Check sheet for the drawn part. Datum: minimum x, y, z corner. Units: mm. A direction names the side the tool comes from. Give positions to 0.01 mm unless a question says otherwise; leave off trailing zeros. Write each loop counter-clockwise with the first axis right and the second up, starting at its lowest first coordinate (ties: lowest second). Pieces come first, ordered by that corner, then holes.
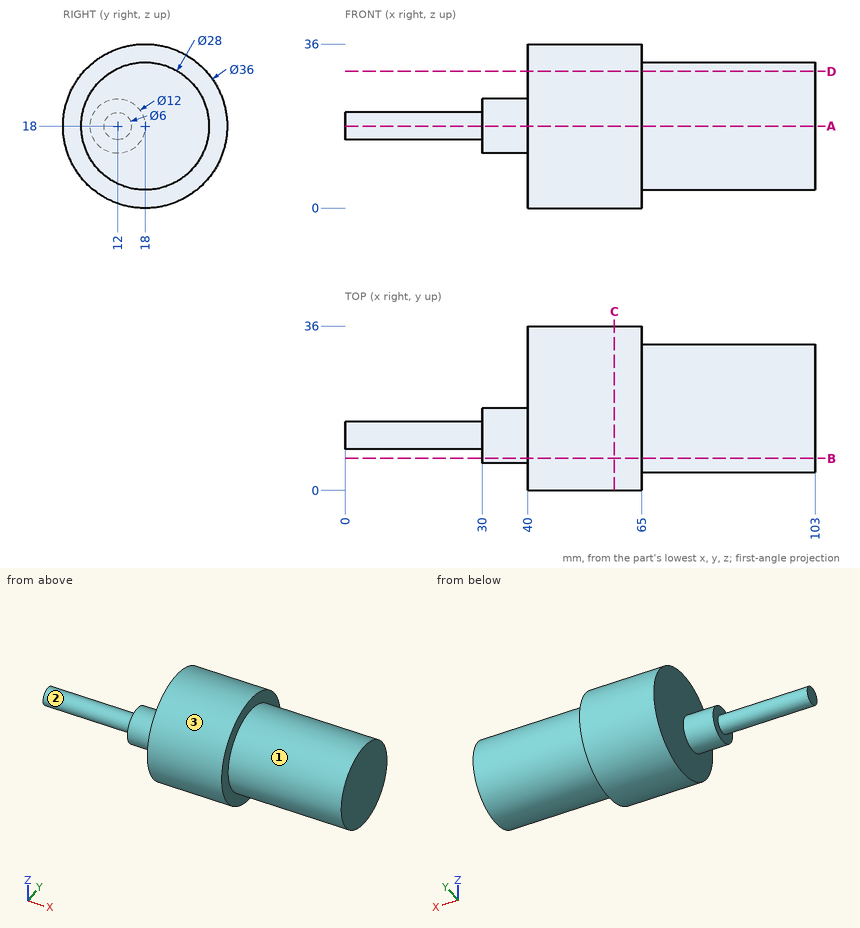
1) Gauge pin test, flat ends, axial feed: pin 1 (12 mm diameter, centred on y = 4.5, z = 6.5, fed in from -X); pin 2 (12 mm diameter, centred on x = 88, y = 32.5, fed in from -Z); pin 3 (1.5 mm diameter, centred on x = 77.5, z = 13, fed in from -Y). Record the tip position at first contact, or that the pin passes through.
2) Sectioned sample at B-B on y = 7. Record the boundary of the cut face in (x, z).
3) Sectioned sample at A-A on z = 18. Record the boundary of the cut face in (x, y), then the cut area to 3 significant figures.
4) Access from +Z, -Z, +X, -X, +Y, -Y to the whole of each face (thin tool, end or side, straight path). Record for the marked faces 1, 2 and 3.
5) Sectioned sample at C-C on x = 59. Record the boundary of the cut face in (y, z).
6) Scan lines: L1, parallel to X at y = 27, z = 10.5; L2, parallel to X at y = 18.5, z = 33.5; L3, parallel to Y at x = 60.5, z = 18. Record each from-to range of solid material in increasing order.
7) Sectioned sample at D-D on z = 30. Record the boundary of the cut face in (x, y).
Answers below:
1. pin 1: stops at x = 40
1. pin 2: stops at z = 6.88
1. pin 3: stops at y = 4.66
2. outline: (30, 14.68) - (40, 14.68) - (40, 3.75) - (65, 3.75) - (65, 9.34) - (103, 9.34) - (103, 26.66) - (65, 26.66) - (65, 32.25) - (40, 32.25) - (40, 21.32) - (30, 21.32) - close
3. outline: (0, 9) - (30, 9) - (30, 6) - (40, 6) - (40, 0) - (65, 0) - (65, 4) - (103, 4) - (103, 32) - (65, 32) - (65, 36) - (40, 36) - (40, 18) - (30, 18) - (30, 15) - (0, 15) - close
3. area: 2,260 mm2
4. face 1: +X
4. face 2: -X
4. face 3: +X, -X
5. outline: circle Ø36 at (18, 18)
6. L1: x = 40 to 103
6. L2: x = 40 to 65
6. L3: y = 0 to 36
7. outline: (40, 4.58) - (65, 4.58) - (65, 10.79) - (103, 10.79) - (103, 25.21) - (65, 25.21) - (65, 31.42) - (40, 31.42) - close
